Part model, mm, in its own coordinate system. Round coordinates to 2 decimals unless told otherwise and drop trailing zeros. Loops run counter-clockwise (first coordinate to the right, second up) from the corner with the lowest first, then second, coordinate; pieces in that order, holes last. Notation, with made-up numbers: (-11, -20.5) -> (41, -20.5) arc R20 ccw to (41, 11.5) -> close; hole circle Ø11 at (54, -35.75). An arc over 180 degrees is marked (long way). Answer as CSV lines item,"result".
from build123d import *

# Parameters (mm, degrees)
CROQUIS1_W            = 16
CROQUIS1_H            = 16
CROQUIS1_W_2          = 14
CROQUIS1_H_2          = 14
EXTRUIR_L_MINA1_DEPTH = 540
CROQUIS2_R            = 2.5
EXTRUIR1_DEPTH        = 541.296215052


with BuildPart() as part:
    # Croquis1 → Extruir-Lámina1 (new, symmetric)
    with BuildSketch(Plane.XY):
        Rectangle(CROQUIS1_W, CROQUIS1_H)
        Rectangle(CROQUIS1_W_2, CROQUIS1_H_2, mode=Mode.SUBTRACT)
    extrude(amount=EXTRUIR_L_MINA1_DEPTH, both=True)

    # Croquis2 → Extruir1 (cut, through all)
    with BuildSketch(Plane(origin=(8, 0, 0), x_dir=(0, 0, -1), z_dir=(1, 0, 0))):
        with Locations((-521, 0)):
            Circle(CROQUIS2_R)
        with Locations(Location((521, 0, 0), (0, 0, 180))):
            Circle(CROQUIS2_R)
    extrude(amount=-EXTRUIR1_DEPTH, mode=Mode.SUBTRACT)


solid = part.part
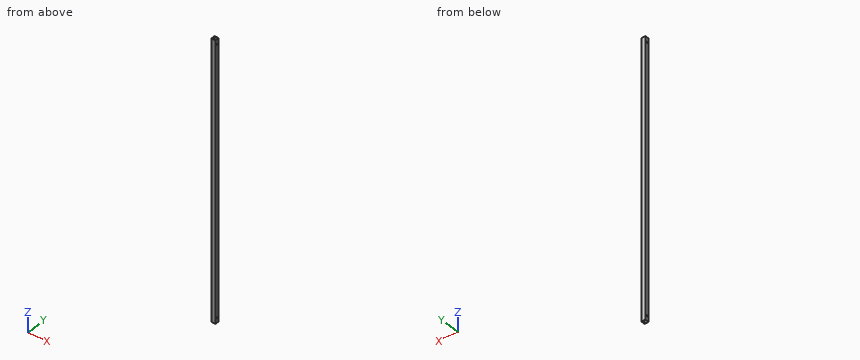
Q1. Saw through at C-C, the plane y = 0. Write the cut outline in (x, z).
Geometry results:
outline,"(-8, -540) -> (-7, -540) -> (-7, -523.5) -> (-8, -523.5) -> close; (-8, -518.5) -> (-7, -518.5) -> (-7, 518.5) -> (-8, 518.5) -> close; (-8, 523.5) -> (-7, 523.5) -> (-7, 540) -> (-8, 540) -> close; (7, -540) -> (8, -540) -> (8, -523.5) -> (7, -523.5) -> close; (7, -518.5) -> (8, -518.5) -> (8, 518.5) -> (7, 518.5) -> close; (7, 523.5) -> (8, 523.5) -> (8, 540) -> (7, 540) -> close"
Q2. Saw through at B-B, the plane z = -238.5. Write the cut outline in (x, y).
Geometry results:
outline,"(-8, -8) -> (8, -8) -> (8, 8) -> (-8, 8) -> close; hole (-7, -7) -> (7, -7) -> (7, 7) -> (-7, 7) -> close"
Q3. Drop a flat-ended pin along its axis: P1, Ø8, axis at x = 2, y = -2.5, coming from the +Z side. Give the stop position or say it passes through.
Geometry results:
P1,"through"
Q4. Drill centre lines: line 1 along Y through (x, z) = (-5.5, -138); line 2 along Y through (x, z) = (-7.4, -521). Where is each one in solid material? Low to high.
Geometry results:
line 1,"-8 to -7, 7 to 8"
line 2,"-8 to -2.5, 2.5 to 8"
Q5. Saw through at A-A, the plane x = 2.5. Write the cut outline in (y, z).
Geometry results:
outline,"(-8, -540) -> (-7, -540) -> (-7, 540) -> (-8, 540) -> close; (7, -540) -> (8, -540) -> (8, 540) -> (7, 540) -> close"
